```python
from build123d import *

# Parameters (mm, degrees)
F0_W     = 149.631724
F0_H     = 198.205128
F1_DEPTH = 25.4
F3_D     = 76.2
F5_D     = 12.7


with BuildPart() as f1:
    # F0 (on Front) → F1 (new body)
    with BuildSketch(Plane.XZ):
        Rectangle(F0_W, F0_H)
    extrude(amount=F1_DEPTH)

    # F3 (through all)
    with Locations(Plane.XZ.offset(25.4)):
        with Locations((0, 0)):
            Hole(F3_D / 2)

    # F5 (through all)
    with Locations(Plane.XZ.offset(25.4)):
        with Locations((0, -59.006654)):
            Hole(F5_D / 2)


solid = f1.part
```
Design review of the part built by this model. Coordinates are the model's own, in mm. Give positions to 0.01 mm unless a question says otherwise; leave off trailing zeros. Loops run counter-clockwise (first coordinate to the right, second up) from the corner with the lowest first, then second, coordinate; pieces in that order, holes last. Notation, with made-up numbers: M -6.5,14 L 5.5,14 A16 cw 5.5,26 Z; hole C -24.75,-25 d7. An arc over 180 degrees is marked long. Return JSON: item names as keys, results as strings. Group by question number.
Item 1: We need section B-B (z = 0). Give the boundary of the cut face in (x, y), and give its area (3 significant figures).
Item 2: We need section C-C (x = 34.5). Give the boundary of the cut face in (y, z), and give its area (3 significant figures).
Item 3: We need section A-A (x = 0). Give the boundary of the cut face in (y, z), and give its area (3 significant figures).
Item 4: For probe 1 along Z at (x, y) = (0, -14.25); probe 2 along Z at (x, y) = (-5, -22.25); probe 3 along X at (y, z) = (-17.75, -62), list the stretches that pass through material, from the lowest coordinate up.
Item 5: We need section D-D (y = -8.25). Give the boundary of the cut face in (x, z).
Item 6: Mouldability with a two-part tool opening along X and no side actions: class faces 1 (the cylindrical face through (0.83, -12.52, -52.71)), 2 (the flat face through (-1, -13, -99.103)), 3 (the flat face through (-74.816, -13, -1)) as released by +X, released by -X, zero draft, split by the parting line, or undercut.
Output:
{
 "1": {"outline": "M -74.82,-25.4 L -38.1,-25.4 L -38.1,0 L -74.82,0 Z; M 38.1,-25.4 L 74.82,-25.4 L 74.82,0 L 38.1,0 Z", "area": "1,870 mm^2"},
 "2": {"outline": "M -25.4,-99.1 L 0,-99.1 L 0,-16.17 L -25.4,-16.17 Z; M -25.4,16.17 L 0,16.17 L 0,99.1 L -25.4,99.1 Z", "area": "4,210 mm^2"},
 "3": {"outline": "M -25.4,-99.1 L 0,-99.1 L 0,-65.36 L -25.4,-65.36 Z; M -25.4,-52.66 L 0,-52.66 L 0,-38.1 L -25.4,-38.1 Z; M -25.4,38.1 L 0,38.1 L 0,99.1 L -25.4,99.1 Z", "area": "2,780 mm^2"},
 "4": {"probe 1": "z = -99.1 to -65.36, -52.66 to -38.1, 38.1 to 99.1", "probe 2": "z = -99.1 to -62.92, -55.09 to -37.77, 37.77 to 99.1", "probe 3": "x = -74.82 to -5.6, 5.6 to 74.82"},
 "5": {"outline": "M -74.82,-99.1 L 74.82,-99.1 L 74.82,99.1 L -74.82,99.1 Z; hole C 0,0 d76.2; hole C 0,-59.01 d12.7"},
 "6": {"face 1": "undercut", "face 2": "zero draft", "face 3": "released by -X"}
}
